Check sheet for the modelled part. Datum: model origin and axes. Units: mm. Face numbers are marked on the shaded views. A direction names the side the tool comes from. Coordinates: 2 decimals unless noted, no trailing zeros. Loops run counter-clockwise (first coordinate to the right, second up) from the corner with the lowest first, then second, coordinate; pieces in that order, holes last. Notation, with made-up numbers: (-6, 83) -> (16, 83) arc R8 cw to (16, 98) -> close; hole circle Ø6 at (-40, 72.5). An arc over 180 degrees is marked (long way). Use one line per item in the form item = value.
from build123d import *

# Parameters (mm, degrees)
BOSS_EXTRUDE1_DEPTH         = 13.89888
CUT_EXTRUDE1_DEPTH          = 69.830593656
CUT_EXTRUDE1_DEPTH_BACK     = 69.830593656
F_1_4_0_25_DIAMETER_HOLE1_D = 6.35


with BuildPart() as part:
    # Sketch1 → Boss-Extrude1 (new body)
    with BuildSketch(Plane(origin=(0, 0, 0), x_dir=(1, 0, 0), z_dir=(0, 1, 0))):
        with BuildLine():
            Line((-53.18125, 6.35), (53.18125, 6.35))
            ThreePointArc((53.18125, 6.35), (65.88125, 0), (53.18125, -6.35))
            Line((53.18125, -6.35), (-53.18125, -6.35))
            ThreePointArc((-53.18125, -6.35), (-65.88125, 0), (-53.18125, 6.35))
        make_face()
    extrude(amount=BOSS_EXTRUDE1_DEPTH)

    # Sketch2 → Cut-Extrude1 (cut, two sides: drawn at the far end of the back side and taken through both)
    with BuildSketch(Plane.XY.offset(6.35).offset(-CUT_EXTRUDE1_DEPTH_BACK)):
        with BuildLine():
            Line((-49.2125, 13.89888), (-36.5125, 13.89888))
            ThreePointArc((-36.5125, 13.89888), (-42.8625, 7.54888), (-49.2125, 13.89888))
        make_face()
        with BuildLine():
            Line((36.5125, 13.89888), (49.2125, 13.89888))
            ThreePointArc((49.2125, 13.89888), (42.8625, 7.54888), (36.5125, 13.89888))
        make_face()
    extrude(amount=CUT_EXTRUDE1_DEPTH + CUT_EXTRUDE1_DEPTH_BACK, mode=Mode.SUBTRACT)

    # 1/4 (0.25) Diameter Hole1 (through all)
    with Locations(Plane(origin=(0, 13.89888, 0), x_dir=(1, 0, 0), z_dir=(0, 1, 0))):
        with Locations((-57.94375, 0), (57.94375, 0)):
            Hole(F_1_4_0_25_DIAMETER_HOLE1_D / 2)


solid = part.part
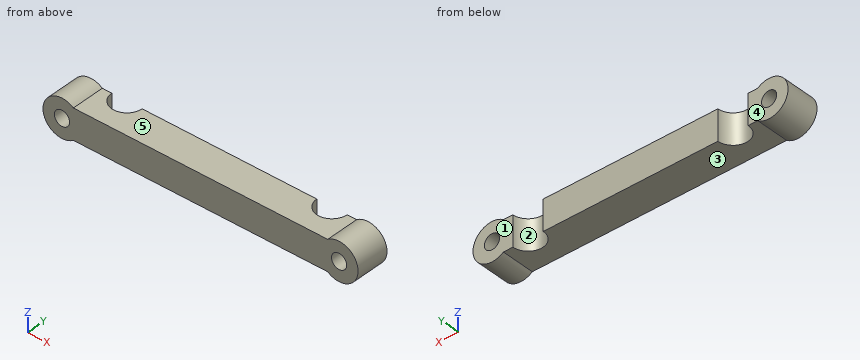
(1) Section check B-B, the plane z = 0. Record the boundary of the cut face in (x, y).
Established:
outline = (-65.88, 0) -> (-61.12, 0) -> (-61.12, 13.9) -> (-65.88, 13.9) -> close; (-54.77, 0) -> (54.77, 0) -> (54.77, 13.9) -> (49.21, 13.9) arc R6.35 cw to (36.51, 13.9) -> (-36.51, 13.9) arc R6.35 cw to (-49.21, 13.9) -> (-54.77, 13.9) -> close; (61.12, 0) -> (65.88, 0) -> (65.88, 13.9) -> (61.12, 13.9) -> close
(2) Section check C-C, the plane z = 5.25. Record the boundary of the cut face in (x, y), plus the area to 3 significant figures.
Established:
outline = (-63.9, 0) -> (63.9, 0) -> (63.9, 13.9) -> (49.21, 13.9) arc R6.35 cw to (36.51, 13.9) -> (-36.51, 13.9) arc R6.35 cw to (-49.21, 13.9) -> (-63.9, 13.9) -> close
area = 1,650 mm²
(3) Section check D-D, the plane x = -6.5. Record the boundary of the cut face in (y, z), plus the area to 3 significant figures.
Established:
outline = (0, -6.35) -> (13.9, -6.35) -> (13.9, 6.35) -> (0, 6.35) -> close
area = 177 mm²
(4) Section check A-A, the plane y = 9.5. Give the number of separate pieces and of enclosed holes in the cut face, plus the area to 3 significant figures.
Established:
separate_pieces = 3
enclosed_holes = 2
area = 1,390 mm²
(5) Scan lines: line 1 along X through (y, z) = (3.25, -0.25); line 2 along Z through (x, y) = (31.5, 5.5); line 3 along X through (y, z) = (4.5, -1). Record each from-to range of solid material in increasing order.
Established:
line_1 = -65.88 to -61.11, -54.78 to 54.78, 61.11 to 65.88
line_2 = -6.35 to 6.35
line_3 = -65.82 to -60.96, -54.93 to 54.93, 60.96 to 65.82
(6) Go/stop test with flat-tipped pins: P1, Ø8.5, axis at x = -57.94, z = 0, coming from the -Y side; P2, Ø8, axis at y = 3.5, z = 5.5, coming from the -X side; P3, Ø3, axis at x = 46.5, y = 5.5, coming from the +Z side; P4, Ø3, axis at y = 4, z = 2.5, coming from the +X side. Record where each tip stops, or that it passes through.
Established:
P1 = 0
P2 = -65.74
P3 = 6.35
P4 = 65.82
(7) Mould release check, pull along X, two halves, no side actions. Record for the marked faces 1 and 2: +X half, -X half, draft (parallel to the pull), parting line (faces both ways), or undercut.
Established:
face_1 = draft
face_2 = undercut
(8) Tool access check on the marked faces 3, 4 and 5. Record the directions out of +Z, -Z, +X, -X, +Y, -Y that give a thin tool (end or side, any length) a straight path to the whole face; none if there is none.
Established:
face_3 = -Z, +Y, -Y
face_4 = +Z, -Z, +X, -X, +Y
face_5 = +Z, +Y, -Y
